Can you work these out from the model? Positions are in its coordinate system, mm. A direction names the side the tool comes from. Coordinates: 2 decimals unless noted, no trailing zeros. Order: outer loops, then holes, each group sorted by start corner. A loop starts at its lowest first (then second) coordinate and runs counter-clockwise, first axis right, second up. Notation, with made-up numbers: M 82.5,21 L 130.5,21 A27 cw 130.5,60 Z; hole C 26,0 d1. An arc over 180 degrees is marked long. Answer as a JSON object with one key per item and string values.
from build123d import *

# Parameters (mm, degrees)
F0_W     = 160
F0_H     = 26
F0_R     = 4
F1_DEPTH = 2
F4_W     = 160
F4_H     = 26
F4_R     = 4
F7_DEPTH = 2
F6_W     = 160
F6_H     = 26
F6_R     = 4
F8_DEPTH = 2
F9_R     = 2


with BuildPart() as f1:
    # F0 (on Top) → F1 (new body)
    with BuildSketch(Plane.XY):
        with Locations((1.2090578675, -20.3812407514)):
            Rectangle(F0_W, F0_H)
        with Locations((-66.7909421325, -20.3812407514)):
            Circle(F0_R, mode=Mode.SUBTRACT)
        with Locations((1.2090578675, -19.4504977352)):
            Circle(F0_R, mode=Mode.SUBTRACT)
        with Locations((69.2090578675, -20.3812407514)):
            Circle(F0_R, mode=Mode.SUBTRACT)
    extrude(amount=F1_DEPTH)

    # F4 (on offset) → F7 (join)
    with BuildSketch(Plane(origin=(0, -7.3812407514, 0), x_dir=(-1, 0, 0), z_dir=(0, 1, 0))):
        with Locations((-1.2090578675, -11)):
            Rectangle(F4_W, F4_H)
        with Locations((-69.2090578675, -11)):
            Circle(F4_R, mode=Mode.SUBTRACT)
        with Locations((-1.2090578675, -11)):
            Circle(F4_R, mode=Mode.SUBTRACT)
        with Locations((66.7909421325, -11)):
            Circle(F4_R, mode=Mode.SUBTRACT)
    extrude(amount=F7_DEPTH)

    # F6 (on offset) → F8 (join)
    with BuildSketch(Plane.XZ.offset(33.3812407514)):
        with Locations((1.2090578675, -11)):
            Rectangle(F6_W, F6_H)
        with Locations((-66.7909421325, -11)):
            Circle(F6_R, mode=Mode.SUBTRACT)
        with Locations((1.2090578675, -11)):
            Circle(F6_R, mode=Mode.SUBTRACT)
        with Locations((69.2090578675, -11)):
            Circle(F6_R, mode=Mode.SUBTRACT)
    extrude(amount=F8_DEPTH)

    # F9
    f9_edges = [f1.edges().sort_by_distance(p)[0] for p in [
        (1.209058, -5.381241, 2),
        (1.209058, -35.381241, 2),
        (-78.790942, -34.381241, -24),
        (-78.790942, -6.381241, -24),
        (81.209058, -34.381241, -24),
        (81.209058, -6.381241, -24),
    ]]
    fillet(f9_edges, radius=F9_R)


solid = f1.part
Item 1: Which directions (+Z, -Z, +X, -X, +Y, -Y) give clear straight access to the entire face, cutting with the end or side of a thin tool? Please do faces 1 (the flat face through (0, -14, 0)), 2 (the cylindrical face through (-70.787, -34.367, -10.824)).
Answers follow:
{"face 1": "-Z, +X, -X", "face 2": "+Y, -Y"}
Item 2: Please list where these lines run through material, in increasing order: line 1 (Y direction, x = -33, z = -1); line 2 (Y direction, x = 0, z = 0.5); line 3 (Z direction, x = 23, y = -12).
Answers follow:
{"line 1": "y = -35.38 to -33.38, -7.38 to -5.38", "line 2": "y = -35.32 to -23.26, -15.64 to -5.44", "line 3": "z = 0 to 2"}
Item 3: If we mould it in two halves opening along X, with no side actions, what happens to faces 3 (the flat face through (81.209, -20, 1)), 4 (the cylindrical face through (73.205, -6.395, -10.824)), 5 (the flat face through (0, -33.381, -17)), 6 (the flat face through (-78.791, -20, 1))? For each: pulls with the +X half, pulls with the -X half, needs draft (parallel to the pull), parting line crosses it, or undercut.
Answers follow:
{"face 3": "pulls with the +X half", "face 4": "undercut", "face 5": "needs draft", "face 6": "pulls with the -X half"}
Item 4: I want a section at D-D, the plane y = -31. Write out the boundary of the cut face in (x, z), plus the area to 3 significant figures.
Answers follow:
{"outline": "M -78.79,0 L 81.21,0 L 81.21,2 L -78.79,2 Z", "area": "320 mm^2"}
Item 5: I'm going to push flat-ended pins straight in: pin 1 (6.5 mm diameter, centred on x = 69.21, z = -11, fed in from +Y); pin 2 (2 mm diameter, centred on x = -19, y = -16.5, fed in from -Z). Where does each tip first touch, or does it pass through?
Answers follow:
{"pin 1": "passes through", "pin 2": "stops at z = 0"}
Item 6: I want a section at B-B, the plane z = -4.25. Write out the boundary of the cut face in (x, y).
Answers follow:
{"outline": "M -78.79,-35.38 L 81.21,-35.38 L 81.21,-33.38 L -78.79,-33.38 Z; M -78.79,-7.38 L 81.21,-7.38 L 81.21,-5.38 L -78.79,-5.38 Z"}
Item 7: I want a section at C-C, the plane x = -51. Write out the boundary of the cut face in (y, z), plus the area to 3 significant figures.
Answers follow:
{"outline": "M -35.38,-24 L -33.38,-24 L -33.38,0 L -7.38,0 L -7.38,-24 L -5.38,-24 L -5.38,0 A2 ccw -7.38,2 L -33.38,2 A2 ccw -35.38,0 Z", "area": "154 mm^2"}
Item 8: I want a section at A-A, the plane z = -11. Give the number of separate pieces and of enclosed holes in the cut face, plus the area to 3 significant figures.
Answers follow:
{"separate pieces": "8", "enclosed holes": "0", "area": "544 mm^2"}
